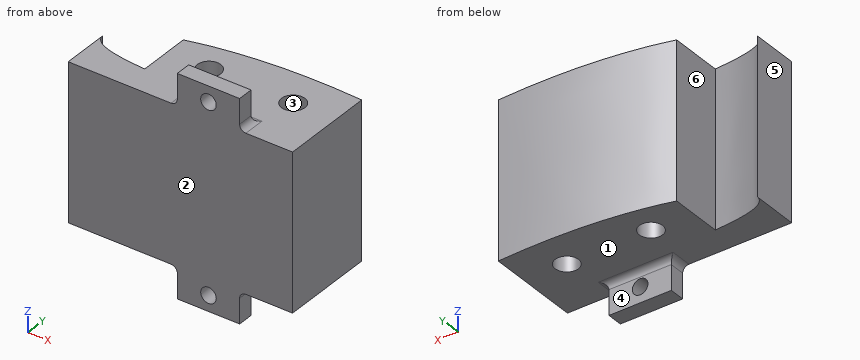
```python
from build123d import *

# Parameters (mm, degrees)
BOSS_EXTRUDE2_DEPTH      = 31.75
BOSS_EXTRUDE2_DEPTH_BACK = 31.75
SKETCH6_R                = 4.7625
SKETCH7_W                = 25.4
SKETCH7_H                = 12.7
SKETCH7_R                = 3.175
BOSS_EXTRUDE3_DEPTH      = 6.35
FILLET2_R                = 2.54


with BuildPart() as part:
    # Sketch6 → Boss-Extrude2 (new, two sides: drawn at the far end of the back side and taken through both)
    with BuildSketch(Plane.XY.offset(-BOSS_EXTRUDE2_DEPTH_BACK)):
        with BuildLine():
            Line((0, 0), (0, -19.05))
            Line((0, -19.05), (91.44, -19.05))
            Line((91.44, -19.05), (91.44, 19.508873689))
            add(Edge.make_bspline(
                [(91.44, 19.508873689), (84.035620806, 19.934056268), (72.792017375, 20.223197155), (57.72640102, 19.576586177), (46.241137994, 18.487194162), (34.713862172, 16.738987134), (26.950784486, 14.94277721), (23.006436851, 13.850652949), (22.86, 13.80984362)],
                knots=[0.299041321, 0.299041321, 0.299041321, 0.299041321, 0.346600594, 0.371102737, 0.395726297, 0.420570145, 0.445825119, 0.446799337, 0.446799337, 0.446799337, 0.446799337], degree=3))
            Line((22.86, 13.80984362), (22.86, -7.674303273))
            add(Edge.make_bspline(
                [(0, 0), (0, -0.17867716), (0.134938936, -1.688448649), (2.416021962, -3.935922156), (6.457030189, -5.50998662), (11.289417386, -6.62752917), (17.013896112, -7.281283102), (20.870897646, -7.562814069), (22.817971884, -7.671962522), (22.86, -7.674303273)],
                knots=[0.505625693, 0.505625693, 0.505625693, 0.505625693, 0.506863029, 0.51614777, 0.522766003, 0.535269014, 0.547551134, 0.559786371, 0.560056294, 0.560056294, 0.560056294, 0.560056294], degree=3))
        make_face()
        with Locations((40.005, 4.734594188)):
            Circle(SKETCH6_R, mode=Mode.SUBTRACT)
        with Locations((74.295, 4.734594188)):
            Circle(SKETCH6_R, mode=Mode.SUBTRACT)
    extrude(amount=BOSS_EXTRUDE2_DEPTH + BOSS_EXTRUDE2_DEPTH_BACK)

    # Sketch7 → Boss-Extrude3 (add)
    # profile 1 of 2: a face of its own
    with BuildSketch(Plane.XZ.offset(19.05)):
        with Locations((57.15, 38.1)):
            Rectangle(SKETCH7_W, SKETCH7_H)
        with Locations(Location((57.15, 38.1, 0), (0, 0, 270))):
            Circle(SKETCH7_R, mode=Mode.SUBTRACT)
    # profile 2 of 2: a face of its own
    with BuildSketch(Plane.XZ.offset(19.05)):
        with Locations((57.15, -38.1)):
            Rectangle(SKETCH7_W, SKETCH7_H)
        with Locations(Location((57.15, -38.1, 0), (0, 0, 90))):
            Circle(SKETCH7_R, mode=Mode.SUBTRACT)
    extrude(amount=-BOSS_EXTRUDE3_DEPTH)

    # Fillet2
    fillet2_edges = [part.edges().sort_by_distance(p)[0] for p in [
        (44.45, -15.875, 31.75),
        (57.15, -12.7, 31.75),
        (69.85, -15.875, 31.75),
        (57.15, -12.7, -31.75),
        (44.45, -15.875, -31.75),
        (69.85, -15.875, -31.75),
    ]]
    fillet(fillet2_edges, radius=FILLET2_R)


solid = part.part
```
Source: CAD feature listing. Evaluate the final solid. Frame: model axes, mm. Face numbers are marked on the shaded views. A direction names the side the tool comes from. Round coordinates to 2 decimals unless told otherwise and drop trailing zeros. Order: outer loops, then holes, each group sorted by start corner. A loop starts at its lowest first (then second) coordinate and runs counter-clockwise, first axis right, second up. Notation, with made-up numbers: (76, 73.5) -> (85, 73.5) arc R19 ccw to (85, 96.5) -> close; hole circle Ø10 at (5, -29). An arc over 180 degrees is marked (long way). Use CSV: the item, a comma, the result in double quotes.
(1) Section B-B on z = 38. Return the cut outline in (x, y), and give its area (3 significant figures).
Report:
outline,"(44.45, -19.05) -> (53.98, -19.05) -> (53.98, -12.7) -> (44.45, -12.7) -> close; (60.32, -19.05) -> (69.85, -19.05) -> (69.85, -12.7) -> (60.32, -12.7) -> close"
area,"121 mm^2"
(2) First-contact query: pin 1 Ø5 at (y, z) = (-17, 37.5) entering from +X; pin 2 Ø15 at (x, y) = (74.3, 4.73) entering from -Z; pin 3 Ø7 at (y, z) = (-14.5, 37) entering from -X; pin 4 Ø7.5 at (x, y) = (40.01, 4.73) entering from -Z. Flat tips, straight axial feed; report the tip coordinate or a pass-through.
Report:
pin 1,"x = 69.85"
pin 2,"z = -31.75"
pin 3,"x = 44.32"
pin 4,"through"
(3) Access query for the marked faces 5 and 6. Directions: +Z, -Z, +X, -X, +Y, -Y. A direction counts if a zero-diameter tool reaches every point of the face in a straight line with its end or side. Return the directions, or none.
Report:
face 5,"+Z, -Z, -X, +Y, -Y"
face 6,"+Z, -Z, +Y"
(4) Section C-C on x = 57.15. Count the separate pieces of the cut face and the enclosed holes in it, and give its area (3 significant figures).
Report:
separate pieces,"3"
enclosed holes,"0"
area,"2,530 mm^2"
(5) Section A-A on z = -38.1. Return the cut outline in (x, y) (3 decimals), and give its area (3 significant figures).
Report:
outline,"(44.45, -19.05) -> (53.975, -19.05) -> (53.975, -12.7) -> (44.45, -12.7) -> close; (60.325, -19.05) -> (69.85, -19.05) -> (69.85, -12.7) -> (60.325, -12.7) -> close"
area,"121 mm^2"
(6) Pull-direction query (Y, two-part tool) for the marked faces 1, 2, 3 and 4; classes: +Y half, -Y half, draft (parallel to the pull), parting line (faces both ways), or undercut.
Report:
face 1,"draft"
face 2,"-Y half"
face 3,"undercut"
face 4,"+Y half"
(7) Ray query, L1, parallel to X at y = 5, z = -9.5; L2, parallel to Z at x = 57, y = -16; L3, parallel to X at y = -17, z = -38. Return the intervals inside material, ascending.
Report:
L1,"22.86 to 35.25, 44.76 to 69.54, 79.05 to 91.44"
L2,"-44.45 to -41.27, -34.93 to 34.93, 41.27 to 44.45"
L3,"44.45 to 53.98, 60.32 to 69.85"
